Autodesk Inventor part; units mm, degrees
ref_plane "YZ Plane" through (0, 0, 0) normal (1, 0, 0) x (0, 1, 0)
ref_plane "XZ Plane" through (0, 0, 0) normal (0, 1, 0) x (-1, 0, 0)
ref_plane "XY Plane" through (0, 0, 0) normal (0, 0, 1) x (1, 0, 0)
sketch "Sketch1" plane through (0, 0, 0) normal (0, 0, 1) x (1, 0, 0)
  circle A0 centre (0, 0) radius 6.35
  circle A1 centre (0, 0) radius 3.175
  line L0 (0, 0) -> (0, 50.8)
  circle A2 centre (0, 50.8) radius 6.35
  circle A3 centre (0, 50.8) radius 3.175
  line L1 (-6.35, 50.8) -> (-6.35, 0)
  line L2 (6.35, 0) -> (6.35, 50.8)
  dimension "d1" = 12.7
  dimension "d2" = 6.35
  dimension "d4" = 50.8
extrude "Extrusion1" add sketch "Sketch1" along normal blind 2.54
properties part number "arm"
Design review of the part built by this model. Coordinates are the model's own, in mm. Coordinates: 2 decimals unless noted, no trailing zeros. Order: outer loops, then holes, each group sorted by start corner. A loop starts at its lowest first (then second) coordinate and runs counter-clockwise, first axis right, second up.
Item 1: Take a section at B-B, the plane y = -2. Write out the cut boundary in (x, z).
Item 2: Take a section at D-D, the plane y = 51.5. Write out the cut boundary in (x, z).
Item 3: The part is to be moulded in two halves that separate along Y. For faces 1 (the cylindrical face through (0.14, -6.35, 1.25)), 2 (the flat face through (0, 26, 0)), 3 (the cylindrical face through (1.707, 48.123, 1.252)), say which applies: pulls with the +Y half, pulls with the -Y half, needs draft (parallel to the pull), parting line crosses it, or undercut.
Item 4: Take a section at C-C, the plane z = 2. Write out the cut boundary in (x, y) (3 decimals), then the cut area to 4 significant figures.
Item 5: Take a section at A-A, the plane x = 0. Write out the cut boundary in (y, z) (3 decimals).
Item 6: For pin 1 Ø1.5 at (x, z) = (5, 0.5) entering from +Y, flat-tipped, find the tip position at first contact; note if it passes through.
Item 7: For line 1 (Y direction, x = 0, z = 1) (3 decimals); line 2 (X direction, y = 50.8, z = 1.4) (3 decimals), list the stretches that pass through material, from the lowest coordinate up.
The answers:
1. outline: (-6.03, 0) - (-2.47, 0) - (-2.47, 2.54) - (-6.03, 2.54) - close; (2.47, 0) - (6.03, 0) - (6.03, 2.54) - (2.47, 2.54) - close
2. outline: (-6.31, 0) - (-3.1, 0) - (-3.1, 2.54) - (-6.31, 2.54) - close; (3.1, 0) - (6.31, 0) - (6.31, 2.54) - (3.1, 2.54) - close
3. face 1: pulls with the -Y half
3. face 2: needs draft
3. face 3: undercut
4. outline: (-6.35, 0) arc R6.35 ccw to (6.35, 0) - (6.35, 50.8) arc R6.35 ccw to (-6.35, 50.8) - close; hole circle Ø6.35 at (0, 0); hole circle Ø6.35 at (0, 50.8)
4. area: 708.5 mm2
5. outline: (-6.35, 0) - (-3.175, 0) - (-3.175, 2.54) - (-6.35, 2.54) - close; (3.175, 0) - (47.625, 0) - (47.625, 2.54) - (3.175, 2.54) - close; (53.975, 0) - (57.15, 0) - (57.15, 2.54) - (53.975, 2.54) - close
6. pin 1: stops at y = 55.52
7. line 1: y = -6.35 to -3.175, 3.175 to 47.625, 53.975 to 57.15
7. line 2: x = -6.35 to -3.175, 3.175 to 6.35
